Design review of the part shown in the three views and the two pictorial views. Dimensions are in mm from the part's minimum x, y and z. Give positions to 0.01 mm unless a question says otherwise; leave off trailing zeros. Write each loop counter-clockwise with the first axis right and the second up, starting at its lowest first coordinate (ties: lowest second). Pieces come first, ordered by that corner, then holes.
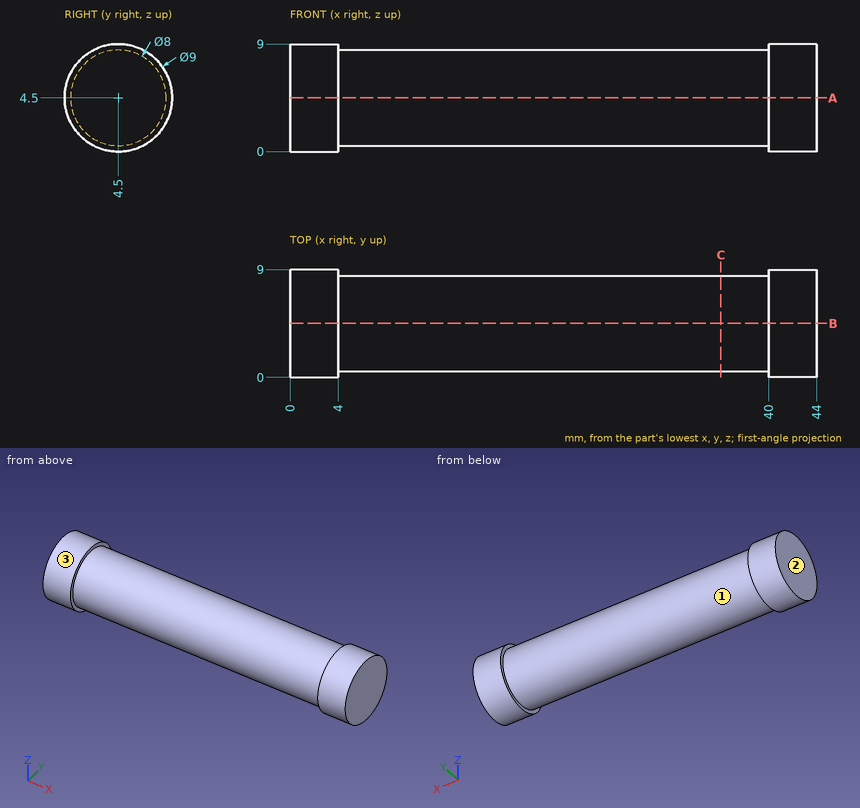
(1) To check wall thickness, follow L1, parallel to X at y = 2.5, z = 1; L2, parallel to Y at x = 2, z = 4.75; L3, parallel to Z at x = 36, y = 5.25. State the ranges of each line that lie inside material, in increasing order.
Resolved:
L1: x = 0 to 4, 40 to 44
L2: y = 0.01 to 8.99
L3: z = 0.57 to 8.43
(2) Mouldability with a two-part tool opening along X and no side actions: class the marked faces 1, 2 and 3 as pulls with the +X half, pulls with the -X half, needs draft (parallel to the pull), parting line crosses it, or undercut.
Resolved:
face 1: undercut
face 2: pulls with the -X half
face 3: needs draft
(3) Consider section A-A, the plane z = 4.5. Give the boundary of the cut face in (x, y), then the cut area to 3 significant figures.
Resolved:
outline: (0, 0) - (4, 0) - (4, 0.5) - (40, 0.5) - (40, 0) - (44, 0) - (44, 9) - (40, 9) - (40, 8.5) - (4, 8.5) - (4, 9) - (0, 9) - close
area: 360 mm2
(4) Clearance check with flat-ended pins moving along their axes: P1, Ø2, axis at x = 28.5, z = 3.5, coming from the -Y side; P2, Ø4.5, axis at y = 4.5, z = 3, coming from the -X side; P3, Ø5, axis at x = 10.5, y = 4, coming from the +Z side. State where each tip first meets the part, or that it passes through.
Resolved:
P1: stops at y = 0.5
P2: stops at x = 0
P3: stops at z = 8.5
(5) Consider section C-C, the plane x = 36. Give the boundary of the cut face in (y, z).
Resolved:
outline: circle Ø8 at (4.5, 4.5)
